Read the model definition and answer for the solid it produces. Units are mm, in the model's axes. Round coordinates to 2 decimals unless told otherwise and drop trailing zeros. Write each loop counter-clockwise with the first axis right and the second up, starting at its lowest first coordinate (ties: lowest second). Pieces come first, ordered by that corner, then holes.
from build123d import *

# Parameters (mm, degrees)
SCHIZZO1_R                   = 2.5
SCHIZZO1_R_2                 = 1.75
ESTRUSIONE_ESTRUSIONE1_DEPTH = 4


with BuildPart() as part:
    # Schizzo1 → Estrusione-Estrusione1 (new body)
    with BuildSketch(Plane.XY):
        with BuildLine():
            Line((0, 0), (0, 449))
            Line((0, 449), (164.5, 449))
            Line((164.5, 449), (164.5, 419))
            ThreePointArc((164.5, 419), (167.428932188, 411.928932188), (174.5, 409))
            Line((174.5, 409), (274.5, 409))
            ThreePointArc((274.5, 409), (281.571067812, 411.928932188), (284.5, 419))
            Line((284.5, 419), (284.5, 449))
            Line((284.5, 449), (449, 449))
            Line((449, 449), (449, 0))
            Line((449, 0), (0, 0))
        make_face()
        with Locations((11.5, 11.5)):
            Circle(SCHIZZO1_R, mode=Mode.SUBTRACT)
        with Locations((437.5, 11.5)):
            Circle(SCHIZZO1_R, mode=Mode.SUBTRACT)
        with Locations((437.5, 437.5)):
            Circle(SCHIZZO1_R, mode=Mode.SUBTRACT)
        with Locations((11.5, 437.5)):
            Circle(SCHIZZO1_R, mode=Mode.SUBTRACT)
        with Locations((319.5, 399)):
            Circle(SCHIZZO1_R_2, mode=Mode.SUBTRACT)
        with BuildLine():
            Line((344.715899345, 409), (405.440355678, 409))
            ThreePointArc((405.440355678, 409), (415.440355678, 399), (405.440355678, 389))
            Line((405.440355678, 389), (344.715899345, 389))
            ThreePointArc((344.715899345, 389), (334.715899345, 399), (344.715899345, 409))
        make_face(mode=Mode.SUBTRACT)
    extrude(amount=ESTRUSIONE_ESTRUSIONE1_DEPTH)


solid = part.part
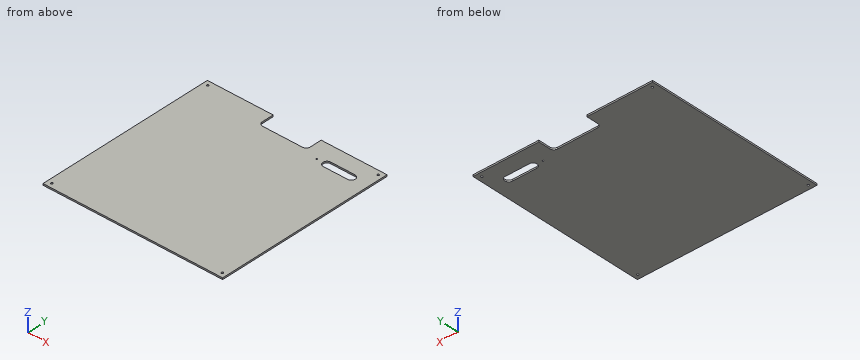
Q1. Section B-B (x = 237.5) is taken. Determine the outline of the cut face in (y, z), then the cut area to 3 significant figures.
Verdict:
outline: (0, 0) - (409, 0) - (409, 4) - (0, 4) - close
area: 1,640 mm2
Q2. Section A-A (z = 1) is taken. Determine the outline of the cut face in (x, y), then the cut area to 3 significant figures.
Verdict:
outline: (0, 0) - (449, 0) - (449, 449) - (284.5, 449) - (284.5, 419) arc R10 cw to (274.5, 409) - (174.5, 409) arc R10 cw to (164.5, 419) - (164.5, 449) - (0, 449) - close; hole circle Ø5 at (11.5, 11.5); hole circle Ø5 at (11.5, 437.5); hole circle Ø3.5 at (319.5, 399); hole (344.72, 389) - (405.44, 389) arc R10 ccw to (405.44, 409) - (344.72, 409) arc R10 ccw to start; hole circle Ø5 at (437.5, 11.5); hole circle Ø5 at (437.5, 437.5)
area: 195,000 mm2
Q3. Straight lines are drawn through the part: probe 1 along X at (y, z) = (399, 0.95); probe 2 along Y at (x, z) = (11.5, 0.85); probe 3 along X at (y, z) = (437.5, 1.6). For each, find the intervals that lie inside material, in ascending order.
Verdict:
probe 1: x = 0 to 317.75, 321.25 to 334.72, 415.44 to 449
probe 2: y = 0 to 9, 14 to 435, 440 to 449
probe 3: x = 0 to 9, 14 to 164.5, 284.5 to 435, 440 to 449
Q4. A flat-ended cylindrical pin translates along its axis: pin 1 Ø2 at (x, z) = (200, 2) entering from +Y. Find the tip coordinate at first contact, or state that the pin passes through.
Verdict:
pin 1: stops at y = 409
